from build123d import *

# Parameters (mm, degrees)
F0_W     = 6.1722
F0_H     = 25.2222
F0_W_2   = 25.5778
F0_H_2   = 6.4389
F1_DEPTH = 6.35


with BuildPart() as f1:
    # F0 (on Top) → F1 (new body)
    with BuildSketch(Plane.XY):
        Polygon((0, 25.4889), (0, 0), (25.3111, 0), (50.8889, 0), (76.1111, 0), (101.6889, 0), (126.9111, 0), (152.4889, 0), (177.8, 0), (177.8, 25.4889), (171.6278, 25.4889), (171.6278, 50.7111), (177.8, 50.7111), (177.8, 76.2), (0, 76.2), (0, 50.7111), (6.1722, 50.7111), (6.1722, 25.4889), align=None)
        with Locations((88.9, 38.1)):
            Rectangle(F0_W, F0_H, mode=Mode.SUBTRACT)
        with Locations((38.1, -3.21945)):
            Rectangle(F0_W_2, F0_H_2)
        with Locations((88.9, -3.21945)):
            Rectangle(F0_W_2, F0_H_2)
        with Locations((139.7, -3.21945)):
            Rectangle(F0_W_2, F0_H_2)
    extrude(amount=F1_DEPTH)


solid = f1.part
Part model, mm, in its own coordinate system. A direction names the side the tool comes from. Give positions to 0.01 mm unless a question says otherwise; leave off trailing zeros. Write each loop counter-clockwise with the first axis right and the second up, starting at its lowest first coordinate (ties: lowest second). Pieces come first, ordered by that corner, then holes.
1) Cut at A-A on y = 34. Write the cut outline in (x, z), then the cut area to 3 significant figures.
Resolved:
outline: (6.17, 0) - (85.81, 0) - (85.81, 6.35) - (6.17, 6.35) - close; (91.99, 0) - (171.63, 0) - (171.63, 6.35) - (91.99, 6.35) - close
area: 1,010 mm2
2) Two-plate mould, pull along Y, no slides. Class faces 1 (the face through (38, -6.439, 3)), 2 (the face through (175, 50.711, 3)), 3 (the face through (88, 54, 6.35)): released by +Y, released by -Y, zero draft, split by the parting line, or undercut.
Resolved:
face 1: released by -Y
face 2: undercut
face 3: zero draft
3) Which spindle directions (+Z, -Z, +X, -X, +Y, -Y) get a long thin tool onto all of the face, cutting with end or side? Do faces 4 (the face through (63, 0, 3)), 5 (the face through (152.489, -3, 3)), 6 (the face through (91.986, 38, 3)), 7 (the face through (171.628, 38, 3)). Say none if no direction does.
Resolved:
face 4: +Z, -Z, -Y
face 5: +Z, -Z, +X, -Y
face 6: +Z, -Z
face 7: +Z, -Z, +X
4) Probe L1, parallel to X at y = 36.5, z = 5.75; L2, parallel to Y at x = 87, z = 1.5; L3, parallel to Y at x = 154.5, z = 4.75. List the from-to ranges inside material, lowest first.
Resolved:
L1: x = 6.17 to 85.81, 91.99 to 171.63
L2: y = -6.44 to 25.49, 50.71 to 76.2
L3: y = 0 to 76.2
5) Pin check, flat tips, straight feed: pin 1 (1.9 mm diameter, centred on x = 4, z = 4, fed in from -Y); pin 2 (3 mm diameter, centred on y = -3.5, z = 2.5, fed in from +X); pin 3 (1.9 mm diameter, centred on y = -3.5, z = 4, fed in from -X). Stop position of each tip, or through.
Resolved:
pin 1: stops at y = 0
pin 2: stops at x = 152.49
pin 3: stops at x = 25.31
6) Cut at C-C on x = 60. Write the cut outline in (y, z), then the cut area to 3 significant figures.
Resolved:
outline: (0, 0) - (76.2, 0) - (76.2, 6.35) - (0, 6.35) - close
area: 484 mm2
7) Cut at B-B on z = 4.75. Write the cut outline in (x, y).
Resolved:
outline: (0, 0) - (25.31, 0) - (25.31, -6.44) - (50.89, -6.44) - (50.89, 0) - (76.11, 0) - (76.11, -6.44) - (101.69, -6.44) - (101.69, 0) - (126.91, 0) - (126.91, -6.44) - (152.49, -6.44) - (152.49, 0) - (177.8, 0) - (177.8, 25.49) - (171.63, 25.49) - (171.63, 50.71) - (177.8, 50.71) - (177.8, 76.2) - (0, 76.2) - (0, 50.71) - (6.17, 50.71) - (6.17, 25.49) - (0, 25.49) - close; hole (85.81, 25.49) - (91.99, 25.49) - (91.99, 50.71) - (85.81, 50.71) - close
